```python
from build123d import *

# Parameters (mm, degrees)
F0_W         = 56
F0_H         = 10
F1_DEPTH     = 1.8
F2_R         = 3
F3_DEPTH     = 10
F4_W         = 10
F4_H         = 10
F5_DEPTH     = 16
F6_W         = 10
F6_H         = 4
F7_DEPTH     = 25
F8_R         = 1.0135034558
F9_DEPTH     = 10
F10_T1_DEPTH = 10
F10_T6_DEPTH = 10
F10_S7_R     = 1.0135034558
F10_T8_DEPTH = 7
F10_T9_DEPTH = 25


# Not quite as in the source:
# - a fillet or chamfer that OpenCascade refuses, or shapes differently, is made with other operations: its cross-section is extruded or revolved along the edge and cut away or added


with BuildPart() as f1:
    # F0 (on Top) → F1 (new body)
    with BuildSketch(Plane.XY):
        Rectangle(F0_W, F0_H)
    extrude(amount=F1_DEPTH)

    # F2
    f2_edges = [f1.edges().sort_by_distance(p)[0] for p in [
        (-28, 5, 0.9),
        (28, 5, 0.9),
        (28, -5, 0.9),
        (-28, -5, 0.9),
    ]]
    fillet(f2_edges, radius=F2_R)

    # F0 (on Top) → F3 (join)
    with BuildSketch(Plane.XY):
        Rectangle(F0_W, F0_H)
    extrude(amount=F3_DEPTH)

    # F4 (on face) → F5 (join)
    with BuildSketch(Plane.XY.offset(10)):
        with Locations((23, 0)):
            Rectangle(F4_W, F4_H)
    extrude(amount=F5_DEPTH)

    # F6 (on face) → F7 (join)
    with BuildSketch(Plane(origin=(18, 0, 0), x_dir=(0, -1, 0), z_dir=(-1, 0, 0))):
        with Locations((0, 24)):
            Rectangle(F6_W, F6_H)
    extrude(amount=F7_DEPTH)

    # F8 (on face) → F9 (cut)
    with BuildSketch(Plane.XY.offset(26)):
        with Locations((-4.0517724119, 0)):
            Circle(F8_R)
        with Locations((-0.6517724119, 0)):
            Circle(F8_R)
        with Locations((2.7482275881, 0)):
            Circle(F8_R)
        with Locations((6.1482275881, 0)):
            Circle(F8_R)
        with Locations((9.5482275881, 0)):
            Circle(F8_R)
        with Locations((12.9482275881, 0)):
            Circle(F8_R)
        with Locations((16.3482275881, 0)):
            Circle(F8_R)
    extrude(amount=-F9_DEPTH, mode=Mode.SUBTRACT)

    # F10: fillet of radius 3 on 6 edges, made by hand

    # F10_s2 → F10_t1 (join)
    with BuildSketch(Plane.XZ.offset(-5)):
        with BuildLine():
            ThreePointArc((18, 13), (17.1213203436, 10.8786796564), (15, 10))
            Line((15, 10), (18, 10))
            Line((18, 10), (18, 13))
        make_face()
    extrude(amount=F10_T1_DEPTH)


with BuildPart() as f10_tool4:
    # F10_s5 → F10_t6 (new body)
    with BuildSketch(Plane.XZ.offset(-5)):
        with BuildLine():
            ThreePointArc((15, 22), (17.1213203436, 21.1213203436), (18, 19))
            Line((18, 19), (18, 22))
            Line((18, 22), (15, 22))
        make_face()
    extrude(amount=F10_T6_DEPTH)

    # F10_s7 → F10_t8 (cut, symmetric)
    with BuildSketch(Plane.XY.offset(20.5)):
        with Locations((16.3482275881, 0)):
            Circle(F10_S7_R)
    extrude(amount=F10_T8_DEPTH, both=True, mode=Mode.SUBTRACT)


with BuildPart() as f1_1:
    add(f1.part)

    # F10_t3: union F10_tool4
    add(f10_tool4.part)

    # F10_s10 → F10_t9 (cut)
    with BuildSketch(Plane.XZ.offset(-12.5)):
        with BuildLine():
            ThreePointArc((25, 26), (27.1213203436, 25.1213203436), (28, 23))
            Line((28, 23), (28, 26))
            Line((28, 26), (25, 26))
        make_face()
        with BuildLine():
            ThreePointArc((28, 3), (27.1213203436, 0.8786796564), (25, 0))
            Line((25, 0), (28, 0))
            Line((28, 0), (28, 3))
        make_face()
        with BuildLine():
            ThreePointArc((-28, 3), (-27.1213203436, 0.8786796564), (-25, 0))
            Line((-25, 0), (-28, 0))
            Line((-28, 0), (-28, 3))
        make_face()
        with BuildLine():
            ThreePointArc((-28, 7), (-27.1213203436, 9.1213203436), (-25, 10))
            Line((-25, 10), (-28, 10))
            Line((-28, 10), (-28, 7))
        make_face()
    extrude(amount=F10_T9_DEPTH, mode=Mode.SUBTRACT)


solid = f1_1.part
```
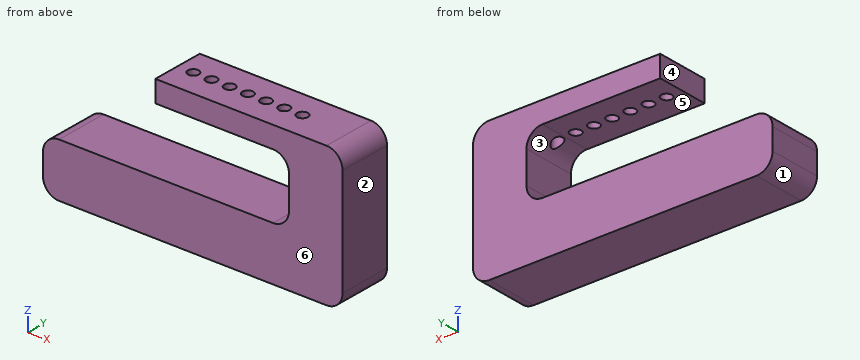
Build history of the part. All positions in model axes, mm. Face numbers are marked on the shaded views. A direction names the side the tool comes from. Give positions to 0.01 mm unless a question says otherwise; leave off trailing zeros. Loops run counter-clockwise (first coordinate to the right, second up) from the corner with the lowest first, then second, coordinate; pieces in that order, holes last. Notation, with made-up numbers: (71.25, 42.25) - (82.25, 42.25) arc R11 ccw to (82.25, 54.25) - close; hole circle Ø6 at (-33.5, 79.25). An arc over 180 degrees is marked (long way). Use a Markdown table: item, result.
(1) Band-saw the part on A-A (y = -2). Give the cut face in (x, z).
Taken from the geometry:
| item | result |
|---|---|
| outline | (-28, 3) arc R3 ccw to (-25, 0) - (25, 0) arc R3 ccw to (28, 3) - (28, 23) arc R3 ccw to (25, 26) - (-7, 26) - (-7, 22) - (15, 22) arc R3 cw to (18, 19) - (18, 13) arc R3 cw to (15, 10) - (-25, 10) arc R3 ccw to (-28, 7) - close |
(2) Wall check: line 1 along Z through (x, y) = (-2, 3.5); line 2 along Z through (x, y) = (-18.5, -1.5); line 3 along X through (y, z) = (4, 19). Give the ranges that are in metal, low to high.
Taken from the geometry:
| item | result |
|---|---|
| line 1 | 0 to 10, 22 to 26 |
| line 2 | 0 to 10 |
| line 3 | 18 to 28 |
(3) Band-saw the part on D-D (x = -21). Give the cut face in (y, z), and give its area (3 significant figures).
Taken from the geometry:
| item | result |
|---|---|
| outline | (-5, 0) - (5, 0) - (5, 10) - (-5, 10) - close |
| area | 100 mm2 |
(4) Drop flat-ended pins along their axis: pin 1 Ø4.5 at (y, z) = (-1.5, 24.5) entering from -X; pin 2 Ø2 at (y, z) = (-4, 14.5) entering from -X; pin 3 Ø1.6 at (x, y) = (9.55, 0) entering from +Z; pin 4 Ø5 at (x, z) = (3, 19) entering from -Y. Give the stop position or say it passes through.
Taken from the geometry:
| item | result |
|---|---|
| pin 1 | x = -7 |
| pin 2 | x = 18 |
| pin 3 | z = 10 |
| pin 4 | through |
(5) Band-saw the part on C-C (x = 13). Give the cut face in (y, z).
Taken from the geometry:
| item | result |
|---|---|
| outline | (-5, 0) - (5, 0) - (5, 10) - (-5, 10) - close; (-5, 22) - (-1.01, 22) - (-1.01, 26) - (-5, 26) - close; (1.01, 22) - (5, 22) - (5, 26) - (1.01, 26) - close |
(6) Pull direction Z, two halves, no side cores. Call the marked faces 1, 2 and 3: +Z half, -Z half, draft (parallel to the pull), parting line (faces both ways), or undercut.
Taken from the geometry:
| item | result |
|---|---|
| face 1 | -Z half |
| face 2 | draft |
| face 3 | undercut |
(7) Band-saw the part on B-B (z = 24). Give the cut face in (x, y), and give its area (3 significant figures).
Taken from the geometry:
| item | result |
|---|---|
| outline | (-7, -5) - (27.83, -5) - (27.83, 5) - (-7, 5) - close; hole circle Ø2.03 at (-4.05, 0); hole circle Ø2.03 at (-0.65, 0); hole circle Ø2.03 at (2.75, 0); hole circle Ø2.03 at (6.15, 0); hole circle Ø2.03 at (9.55, 0); hole circle Ø2.03 at (12.95, 0); hole circle Ø2.03 at (16.35, 0) |
| area | 326 mm2 |
(8) Which spindle directions (+Z, -Z, +X, -X, +Y, -Y) get a long thin tool onto all of the face, cutting with end or side? Do the marked faces 4, 5 and 6. Say none if no direction does.
Taken from the geometry:
| item | result |
|---|---|
| face 4 | +Z, -X, +Y, -Y |
| face 5 | -X, +Y, -Y |
| face 6 | +Z, -Z, +X, -X, -Y |
